Build history of the part. All positions in model axes, mm. Round coordinates to 2 decimals unless told otherwise and drop trailing zeros. Loops run counter-clockwise (first coordinate to the right, second up) from the corner with the lowest first, then second, coordinate; pieces in that order, holes last. Notation, with made-up numbers: (-1.75, -24) -> (48.25, -24) arc R23 ccw to (48.25, 10) -> close; hole circle Ø5 at (3.25, 52.5). An arc over 180 degrees is marked (long way). Put each result on its own line as item: value. Start each with the question number.
Item 1: Cut at B-B, the plane y = 104. List the corners of the cut face in (x, z).
Item 2: Flat gauge pin, fed straight in: pin 1 Ø4 at (x, y) = (-37.5, 74) entering from +Z (3 decimals). Where does the tip first touch, or does it go through?
Item 3: Cut at A-A, the plane x = -50. List the corners of the cut face in (y, z).
Item 4: Drill centre lines: probe 1 along Y at (x, z) = (-37.5, 3); probe 2 along Y at (x, z) = (25, 4.5); probe 3 along Y at (x, z) = (-20, 4.5). Where is each one in solid material? Low to high. Write a range as [from, to].
Item 5: Cut at C-C, the plane z = 4. Count the separate pieces of the cut face and the enclosed holes in it, plus the area to 3 significant figures.
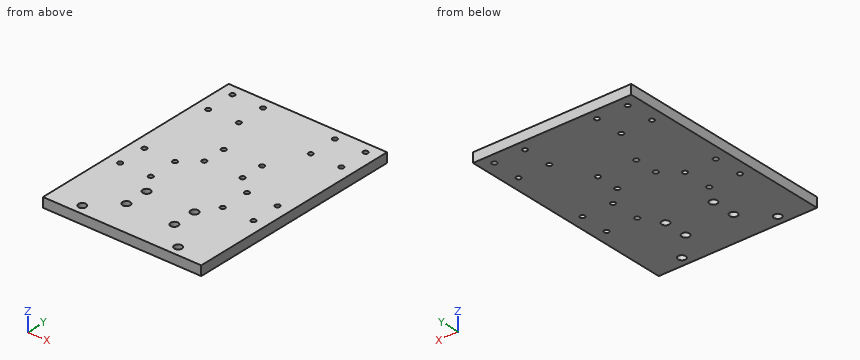
```python
from build123d import *

# Parameters (mm, degrees)
SKETCH1_W           = 165
SKETCH1_H           = 230
BOSS_EXTRUDE1_DEPTH = 10
OTW_R_5_0_5_1_D     = 5
OTW_R_8_0_8_1_D     = 8
OTW_R_8_0_8_2_D     = 8


with BuildPart() as part:
    # Sketch1 → Boss-Extrude1 (new body)
    with BuildSketch(Plane.XY):
        Rectangle(SKETCH1_W, SKETCH1_H)
    extrude(amount=BOSS_EXTRUDE1_DEPTH)

    # Otwór Ø5.0 (5)1 (through all)
    with Locations(Plane(origin=(0, 0, 0), x_dir=(-1, 0, 0), z_dir=(0, 0, -1))):
        with Locations((-69.5, 104), (-37.5, 104), (-37.5, 74), (-69.5, 74), (-69.5, -5), (-37.5, -5), (-37.5, -35), (-69.5, -35), (37.5, 104), (69.5, 104), (69.5, 74), (37.5, 74), (37.5, -5), (69.5, -5), (69.5, -35), (37.5, -35), (-20, 34.5), (20, 34.5), (20, 10.5), (-20, 10.5)):
            Hole(OTW_R_5_0_5_1_D / 2)

    # Otwór Ø8.0 (8)1 (through all)
    with Locations(Plane.XY.offset(10)):
        with Locations((-25, -55), (25, -55), (25, -80), (-25, -80)):
            Hole(OTW_R_8_0_8_1_D / 2)

    # Otwór Ø8.0 (8)2 (through all)
    with Locations(Plane.XY.offset(10)):
        with Locations((50, -105), (-50, -105)):
            Hole(OTW_R_8_0_8_2_D / 2)


solid = part.part
```
Reply:
1. outline: (-82.5, 0) -> (-72, 0) -> (-72, 10) -> (-82.5, 10) -> close; (-67, 0) -> (-40, 0) -> (-40, 10) -> (-67, 10) -> close; (-35, 0) -> (35, 0) -> (35, 10) -> (-35, 10) -> close; (40, 0) -> (67, 0) -> (67, 10) -> (40, 10) -> close; (72, 0) -> (82.5, 0) -> (82.5, 10) -> (72, 10) -> close
2. pin 1: passes through
3. outline: (-115, 0) -> (-109, 0) -> (-109, 10) -> (-115, 10) -> close; (-101, 0) -> (115, 0) -> (115, 10) -> (-101, 10) -> close
4. probe 1: y = [-115, -37.5], [-32.5, -7.5], [-2.5, 71.5], [76.5, 101.5], [106.5, 115]
4. probe 2: y = [-115, -84], [-76, -59], [-51, 115]
4. probe 3: y = [-115, 8], [13, 32], [37, 115]
5. separate pieces: 1
5. enclosed holes: 26
5. area: 37,300 mm^2
